Geometry check sheet. Reference: drawing and pictorial views, mm from the part's lowest x, y, z. A direction names the side the tool comes from. Give positions to 0.01 mm unless a question says otherwise; leave off trailing zeros. Loops run counter-clockwise (first coordinate to the right, second up) from the corner with the lowest first, then second, coordinate; pieces in that order, holes last. Notation, with made-up numbers: (3.5, 40) - (32.5, 40) arc R10 cw to (32.5, 50) - close; hole circle Ø3 at (22.25, 37.25). An arc over 180 degrees is marked (long way). One line per question, with ' | ' between items. Start each with the question number.
1. Tool access check on the marked faces 1 and 2. Record the directions out of +Z, -Z, +X, -X, +Y, -Y that give a thin tool (end or side, any length) a straight path to the whole face; none if there is none.
2. Thickness scan on line 1 along Z through (x, y) = (2, 20); line 2 along X through (y, z) = (18, 7.5) (1 decimal); line 3 along X through (y, z) = (10, 7) (1 decimal). Record the ranges inside material, lowest first. Write a range as from..to.
3. Mould release check, pull along X, two halves, no side actions. Record for the marked faces 3, 4 and 5: +X half, -X half, draft (parallel to the pull), parting line (faces both ways), or undercut.
4. Section check B-B, the plane z = 4.75. Enter the section's corners in (x, y) (1 decimal).
5. Section check D-D, the plane y = 23. Enter the section's corners in (x, z), then the cut area to 3 significant figures.
6. Depth check by flat-ended pin: pin 1 Ø3.5 at (x, z) = (17, 4.5) entering from -Y; pin 2 Ø3 at (x, z) = (24, 3) entering from -Y; pin 3 Ø1 at (y, z) = (26.5, 3.5) entering from -X (1 decimal). Enter the tip coordinate at first touch or a pass-through.
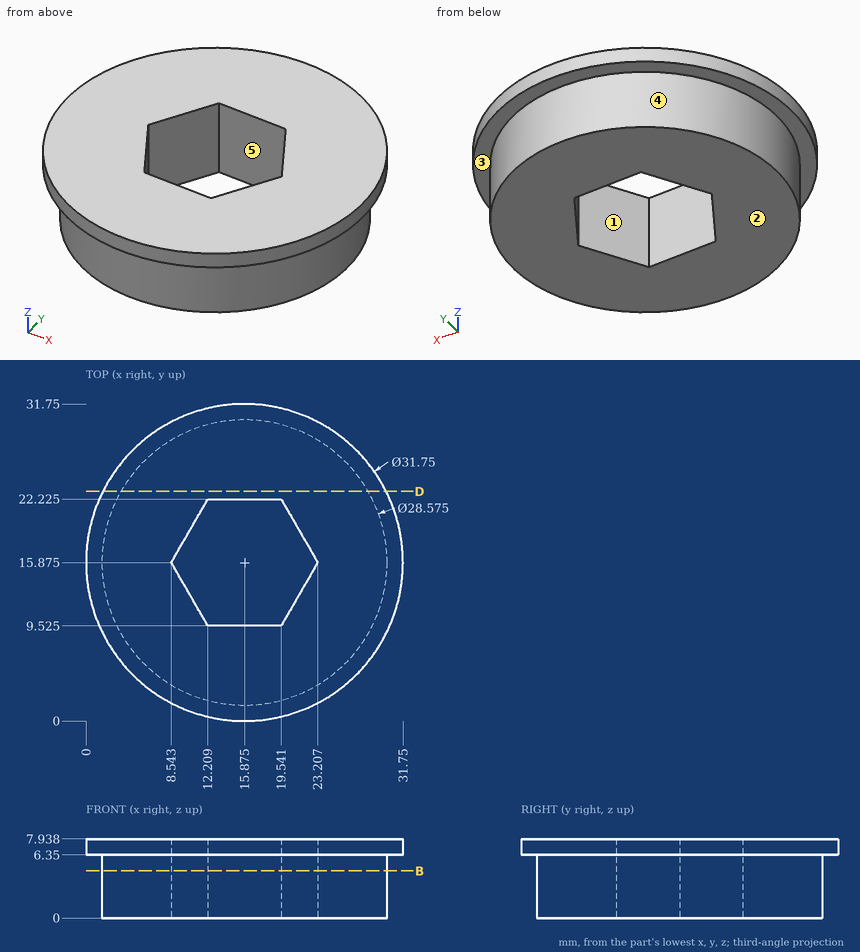
Results list:
1) face 1: +Z, -Z | face 2: -Z, +X, -X, +Y, -Y
2) line 1: 6.35..7.94 | line 2: 0.1..9.8, 22..31.6 | line 3: 1.1..11.9, 19.8..30.6
3) face 3: draft | face 4: parting line | face 5: undercut
4) outline: circle Ø28.6 at (15.9, 15.9); hole (8.5, 15.9) - (12.2, 9.5) - (19.5, 9.5) - (23.2, 15.9) - (19.5, 22.2) - (12.2, 22.2) - close
5) outline: (1.69, 6.35) - (3.49, 6.35) - (3.49, 0) - (28.26, 0) - (28.26, 6.35) - (30.06, 6.35) - (30.06, 7.94) - (1.69, 7.94) - close | area: 202 mm²
6) pin 1: y = 1.59 | pin 2: y = 3.22 | pin 3: x = 5.8
